Geometry check sheet. Reference: the model listing, model coordinates, mm. A direction names the side the tool comes from. Give positions to 0.01 mm unless a question says otherwise; leave off trailing zeros. Write each loop counter-clockwise with the first axis right and the second up, starting at its lowest first coordinate (ties: lowest second). Pieces come first, ordered by that corner, then holes. Notation, with made-up numbers: (-6, 36.5) - (49, 36.5) arc R24 cw to (49, 46.5) - close; hole circle Ø7 at (11, 31). An arc over 180 degrees is marked (long way). Write item = value, one per line. Start each with the question number.
(1) Thickness scan on L1, parallel to Y at x = 0, z = 17; L2, parallel to X at y = -17.5, z = 53; L3, parallel to Y at x = -14.5, z = 75.5. Record the ranges inside material, lowest first.
(2) Section check A-A, the plane x = 0. Enter the section's corners in (y, z), plus the area to 3 significant figures.
(3) Section check B-B, the plane z = 65.5. Enter the section's corners in (x, y).
(4) Draft check along X on faces 3 (the cylindrical face through (47.69, 15.02, 39.96)), 4 (the cylindrical face through (-1.172, 8.923, 20.009)), 5 (the flat face through (-22.5, 11.6, 80)). Enter one of: pulls with the +X half, pulls with the -X half, needs draft (parallel to the pull), parting line crosses it, or undercut.
(5) Access from +Z, -Z, +X, -X, +Y, -Y to the whole of each face (thin tool, end or side, straight path). Record for faces 1 (the flat face through (21.75, 12.33, 64.11)), 2 (the flat face through (-0.7, 11.3, 0)).
(6) Depth check by flat-ended pin: pin 1 Ø4 at (x, y) = (9.5, 15) entering from +Z; pin 2 Ø1 at (y, z) = (27, 37.5) entering from -X; pin 3 Ø6 at (x, z) = (-31, 25) entering from -Y. Enter the tip coordinate at first touch or a pass-through.
```python
from build123d import *

# Parameters (mm, degrees)
SKIZZE1_R                       = 50
SKIZZE1_R_2                     = 9
AUFSATZ_LINEAR_AUSTRAGEN1_DEPTH = 80
VERRUNDUNG1_R                   = 2
VERRUNDUNG2_R                   = 1
AUFSATZ_LINEAR_AUSTRAGEN2_DEPTH = 30
SKIZZE12_OUTSIDE_W              = 134.496
SKIZZE12_OUTSIDE_H              = 134.496
SCHNITT_LINEAR_AUSTRAGEN3_DEPTH = 81


with BuildPart() as part:
    # Skizze1 → Aufsatz-Linear austragen1 (new body)
    with BuildSketch(Plane.XY):
        Circle(SKIZZE1_R)
        Circle(SKIZZE1_R_2, mode=Mode.SUBTRACT)
    extrude(amount=AUFSATZ_LINEAR_AUSTRAGEN1_DEPTH)

    # Verrundung1
    verrundung1_edges = [part.edges().sort_by_distance(p)[0] for p in [
        (-50, 0, 0),
        (-9, 0, 0),
    ]]
    fillet(verrundung1_edges, radius=VERRUNDUNG1_R)

    # Verrundung2
    verrundung2_edges = [part.edges().sort_by_distance(p)[0] for p in [
        (-50, 0, 80),
    ]]
    fillet(verrundung2_edges, radius=VERRUNDUNG2_R)


with BuildPart() as body_2:
    # Skizze2 → Aufsatz-Linear austragen2 (new body)
    with BuildSketch(Plane.XY.offset(80)):
        Polygon((28.867513459, 0), (14.43375673, 25), (-14.43375673, 25), (-28.867513459, 0), (-14.43375673, -25), (14.43375673, -25), align=None)
    extrude(amount=-AUFSATZ_LINEAR_AUSTRAGEN2_DEPTH)

    # Skizze10 → Rotation1 (revolve)
    with BuildSketch(Plane(origin=(-14.43375673, 0, 0), x_dir=(0, 0, 1), z_dir=(0, -1, 0)), mode=Mode.PRIVATE) as rotation1_sk:
        Polygon((50, 14.43375673), (33.333333333, -14.43375673), (50, -14.43375673), align=None)
    revolve(rotation1_sk.sketch.rotate(Axis((0, 0, 33.333333333), (0, 0, 1)), 180), axis=Axis((0, 0, 33.333333333), (0, 0, 1)))  # turned: the seam where the file's is

    # Skizze12 outside → Schnitt-Linear austragen3 (cut, through all)
    with BuildSketch(Plane.XY.offset(80)):
        Rectangle(SKIZZE12_OUTSIDE_W, SKIZZE12_OUTSIDE_H)
        Polygon((14.43375673, -25), (28.867513459, 0), (14.43375673, 25), (-14.43375673, 25), (-28.867513459, 0), (-14.43375673, -25), align=None, mode=Mode.SUBTRACT)
    extrude(amount=-SCHNITT_LINEAR_AUSTRAGEN3_DEPTH, mode=Mode.SUBTRACT)


with BuildPart() as part_1:
    add(part.part)

    # Kombinieren1: cut body 2
    add(body_2.part, mode=Mode.SUBTRACT)


solid = part_1.part
```
Model answer:
q1.L1 = -50 to -9, 9 to 50
q1.L2 = -46.84 to -18.76, 18.76 to 46.84
q1.L3 = -47.85 to -24.89, 24.89 to 47.85
q2.outline = (-50, 2) arc R2 ccw to (-48, 0) - (-11, 0) arc R2 ccw to (-9, 2) - (-9, 38.53) - (-25, 47.77) - (-25, 80) - (-49, 80) arc R1 ccw to (-50, 79) - close; (9, 2) arc R2 ccw to (11, 0) - (48, 0) arc R2 ccw to (50, 2) - (50, 79) arc R1 ccw to (49, 80) - (25, 80) - (25, 47.77) - (9, 38.53) - close
q2.area = 5,380 mm²
q3.outline = circle Ø100 at (0, 0); hole (-28.87, 0) - (-14.43, -25) - (14.43, -25) - (28.87, 0) - (14.43, 25) - (-14.43, 25) - close
q4.face_3 = parting line crosses it
q4.face_4 = undercut
q4.face_5 = needs draft
q5.face_1 = +Z
q5.face_2 = -Z, +X, -X, +Y, -Y
q6.pin_1 = 44.74
q6.pin_2 = -42.4
q6.pin_3 = -41.42
